Read the model definition and answer for the solid it produces. Units are mm, in the model's axes. Face numbers are marked on the shaded views. Coordinates: 2 decimals unless noted, no trailing zeros. Order: outer loops, then holes, each group sorted by start corner. A loop starts at its lowest first (then second) coordinate and runs counter-clockwise, first axis right, second up. Notation, with made-up numbers: (39, -7) -> (52, -7) arc R27 ccw to (52, 20) -> close; hole circle Ø5 at (-22.5, 38). An arc over 180 degrees is marked (long way). Answer in a Markdown table with one row per item.
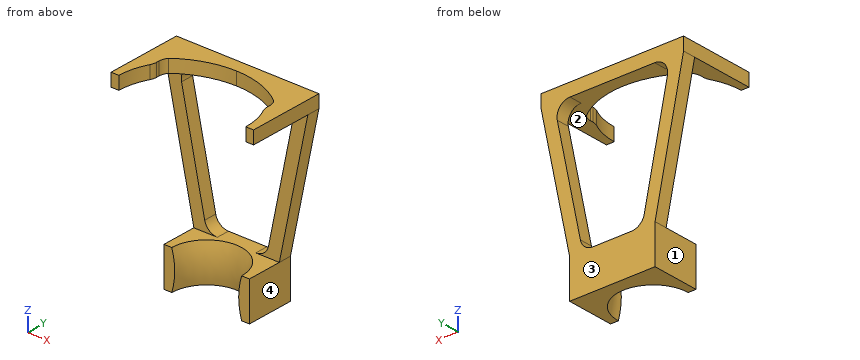
from build123d import *

# Parameters (mm, degrees)
BOSS_EXTRUDE1_DEPTH = 5
BOSS_EXTRUDE2_START = -53
BOSS_EXTRUDE2_DEPTH = 15
REVOLVE2_ANGLE      = 180
BOSS_EXTRUDE3_DEPTH = 5
FILLET1_R           = 5


with BuildPart() as part:
    # Sketch1 → Boss-Extrude1 (new body)
    with BuildSketch(Plane.XY):
        with BuildLine():
            Line((-21.323076923, 14.485250559), (-21.323076923, 13.317117605))
            ThreePointArc((-21.323076923, 13.317117605), (-21.459554932, 12.156878903), (-21.861538462, 11.059979028))
            ThreePointArc((-21.861538462, 11.059979028), (-23.831257754, 5.685169641), (-24.5, 0))
            Line((-24.5, 0), (-27.5, 0))
            Line((-27.5, 0), (-27.5, 29.5))
            Line((-27.5, 29.5), (27.5, 29.5))
            Line((27.5, 29.5), (27.5, 0))
            Line((27.5, 0), (24.5, 0))
            ThreePointArc((24.5, 0), (23.831257754, 5.685169641), (21.861538462, 11.059979028))
            ThreePointArc((21.861538462, 11.059979028), (21.459554932, 12.156878903), (21.323076923, 13.317117605))
            Line((21.323076923, 13.317117605), (21.323076923, 14.485250559))
            ThreePointArc((21.323076923, 14.485250559), (21.059553746, 16.08705807), (20.296762002, 17.52002022))
            ThreePointArc((20.296762002, 17.52002022), (10.731713115, 22.70625472), (0, 24.5))
            ThreePointArc((0, 24.5), (-10.731713115, 22.70625472), (-20.296762002, 17.52002022))
            ThreePointArc((-20.296762002, 17.52002022), (-21.059553746, 16.08705807), (-21.323076923, 14.485250559))
        make_face()
    extrude(amount=BOSS_EXTRUDE1_DEPTH)



with BuildPart() as body_2:
    # Sketch2 → Boss-Extrude2 (new body)
    with BuildSketch(Plane.XY.offset(BOSS_EXTRUDE2_START)):
        with BuildLine():
            Line((-16.5, 11), (-13.5, 11))
            ThreePointArc((-13.5, 11), (0, 24.5), (13.5, 11))
            Line((13.5, 11), (16.5, 11))
            Line((16.5, 11), (16.5, 29.5))
            Line((16.5, 29.5), (-16.5, 29.5))
            Line((-16.5, 29.5), (-16.5, 11))
        make_face()
    extrude(amount=-BOSS_EXTRUDE2_DEPTH)

    # Sketch5 → Revolve2 (revolve)
    with BuildSketch(Plane.XZ.offset(-11)):
        with BuildLine():
            Line((13.5, -53), (13.5, -68))
            ThreePointArc((13.5, -68), (12.348480035, -60.5), (13.5, -53))
        make_face()
    revolve(axis=Axis((0, 11, -60.5), (0, 0, 1)), revolution_arc=REVOLVE2_ANGLE)


with BuildPart() as part_1:
    add(part.part)

    add(body_2.part)  # Boss-Extrude3 merges body 2
    # Sketch6 → Boss-Extrude3 (add)
    with BuildSketch(Plane(origin=(0, 29.5, 0), x_dir=(1, 0, 0), z_dir=(0, 1, 0))):
        Polygon((-27.5, 0), (-16.5, 53), (-11.5, 53), (-22.5, 0), align=None)
        Polygon((22.5, 0), (11.5, 53), (16.5, 53), (27.5, 0), align=None)
    extrude(amount=-BOSS_EXTRUDE3_DEPTH)

    # Fillet1
    fillet1_edges = [part_1.edges().sort_by_distance(p)[0] for p in [
        (-22.5, 27, 0),
        (-11.5, 27, -53),
        (22.5, 27, 0),
        (11.5, 27, -53),
    ]]
    fillet(fillet1_edges, radius=FILLET1_R)


solid = part_1.part
Q1. The part is cut by section C-C (z = -1.5). Write down the section's boundary in (x, y), then the cut area to 3 significant figures.
Outcome:
| item | result |
|---|---|
| outline | (-27.19, 24.5) -> (-19.93, 24.5) -> (-19.93, 29.5) -> (-27.19, 29.5) -> close; (19.93, 24.5) -> (27.19, 24.5) -> (27.19, 29.5) -> (19.93, 29.5) -> close |
| area | 72.6 mm² |
Q2. Consider line 1 (Z direction, x = 4, y = 25.25); line 2 (Z direction, x = 14, y = 19.5); line 3 (Y direction, x = -18.5, z = -39). Determine where each line is inside the solid, lowest interval first.
Outcome:
| item | result |
|---|---|
| line 1 | -68 to -53, 0 to 5 |
| line 2 | -68 to -53 |
| line 3 | 24.5 to 29.5 |
Q3. The part is cut by section D-D (z = -55). Write down the section's boundary in (x, y), then the cut area to 3 significant figures.
Outcome:
| item | result |
|---|---|
| outline | (-16.5, 11) -> (-12.96, 11) arc R12.96 cw to (12.96, 11) -> (16.5, 11) -> (16.5, 29.5) -> (-16.5, 29.5) -> close |
| area | 347 mm² |
Q4. The part is cut by section A-A (y = 8). Write down the section's boundary in (x, z).
Outcome:
| item | result |
|---|---|
| outline | (-27.5, 0) -> (-23.16, 0) -> (-23.16, 5) -> (-27.5, 5) -> close; (23.16, 0) -> (27.5, 0) -> (27.5, 5) -> (23.16, 5) -> close |
Q5. For a pull along X with two mould halves and no side action, classify the marked faces 1, 2, 3 and 4 as pulls with the +X half, pulls with the -X half, needs draft (parallel to the pull), parting line crosses it, or undercut.
Outcome:
| item | result |
|---|---|
| face 1 | pulls with the -X half |
| face 2 | undercut |
| face 3 | needs draft |
| face 4 | pulls with the +X half |
Q6. Given pin 1 (4 mm diameter, centred on x = 16.5, y = 9.5, fed in from +Z); pin 2 (1.2 mm diameter, centred on x = -14.5, z = -60, fed in from -Y); pin 3 (5 mm diameter, centred on y = 16.5, z = -56.5, fed in from -X), each flat-ended and moving along its own axis, determine where each tip first touches the part or whether it passes through.
Outcome:
| item | result |
|---|---|
| pin 1 | z = -53 |
| pin 2 | y = 11 |
| pin 3 | x = -16.5 |
Q7. The part is cut by section B-B (x = -15.5). Write down the section's boundary in (y, z).
Outcome:
| item | result |
|---|---|
| outline | (11, -68) -> (29.5, -68) -> (29.5, -33.73) -> (24.5, -33.73) -> (24.5, -53) -> (11, -53) -> close; (20.63, 0) -> (29.5, 0) -> (29.5, 5) -> (20.63, 5) -> close |
